Could you check a few things on this model? Use its own coordinates, in mm. Give positions to 0.01 mm unless a question says otherwise; leave off trailing zeros. Write each loop counter-clockwise with the first axis right and the second up, starting at its lowest first coordinate (ties: lowest second). Pieces come first, ordered by that corner, then holes. Notation, with made-up numbers: (60, 6) -> (86, 6) arc R16 ccw to (86, 13) -> close; hole circle Ø5 at (56.25, -27.5). An arc over 180 degrees is marked (long way). One line per question, with ' | ' between items.
from build123d import *

# Parameters (mm, degrees)
BLANKSKE_W              = 126
BLANKSKE_H              = 26.5
BLANK_DEPTH             = 6
TOOTHCUTSIM_DEPTH       = 129.896276129
TEETHCUTS_COUNT         = 33
TEETHCUTS_PITCH         = 4.712388975
ESQUISSE1_R             = 1.25
ENL_V_MAT_EXTRU_1_DEPTH = 6


with BuildPart() as part:
    # BlankSke → Blank (new body)
    with BuildSketch(Plane.XY):
        with Locations((63, 13.25)):
            Rectangle(BLANKSKE_W, BLANKSKE_H)
    extrude(amount=-BLANK_DEPTH)

    # TooCutSkeSim → ToothCutSim (cut, through all)
    with BuildSketch(Plane.XY):
        Polygon((0.654653055, 23.125), (-0.654653055, 23.125), (-1.892297439, 26.5254), (1.892297439, 26.5254), align=None)
    toothcutsim = extrude(amount=-TOOTHCUTSIM_DEPTH, mode=Mode.SUBTRACT)

    # TeethCuts: ToothCutSim ×33
    with Locations(*[(i * TEETHCUTS_PITCH, 0, 0) for i in range(1, TEETHCUTS_COUNT)]):
        add(toothcutsim, mode=Mode.SUBTRACT)

    # Esquisse1 → Enlèv. mat.-Extru.1 (cut)
    with BuildSketch(Plane.XY):
        with Locations((5, 11.5)):
            Circle(ESQUISSE1_R)
        with Locations((25, 11.5)):
            Circle(ESQUISSE1_R)
    extrude(amount=-ENL_V_MAT_EXTRU_1_DEPTH, mode=Mode.SUBTRACT)


solid = part.part
Q1. Imagine slicing it at A-A on y = 11.5. Please give me the cut outline in (x, z).
Answer below:
outline: (0, -6) -> (3.75, -6) -> (3.75, 0) -> (0, 0) -> close; (6.25, -6) -> (23.75, -6) -> (23.75, 0) -> (6.25, 0) -> close; (26.25, -6) -> (126, -6) -> (126, 0) -> (26.25, 0) -> close
Q2. Will this pin go through, and if not, where does the flat tip stop? pin 1 (1 mm diameter, centred on x = 47, z = -3, fed in from +Y) (3 decimals).
Answer below:
pin 1: stops at y = 23.125
Q3. If I drill on line 1 along Y through (x, z) = (13.5, -2.95) (3 decimals), over which ranges is the centre line in solid material (lowest first)?
Answer below:
line 1: y = 0 to 23.125
Q4. Imagine slicing it at B-B on z = -4.7. Count the separate pieces of the cut face and the enclosed holes in it, and give its area (3 significant figures).
Answer below:
separate pieces: 1 | enclosed holes: 2 | area: 3,100 mm^2
Q5. If we mould it in two halves opening along X, with no side actions, what happens to faces 1 (the flat face through (62, 10, -6)), 2 (the flat face through (0, 11, -3)), 3 (the flat face through (123.8, 24.84, -2.96))? For each: +X half, -X half, draft (parallel to the pull), parting line (faces both ways), or undercut.
Answer below:
face 1: draft | face 2: -X half | face 3: undercut
